Autodesk Fusion 360 part; units mm, degrees
sketch "Sketch1" plane through (0, 0, 0) normal (0, 0, 1) x (1, 0, 0)
  line L0 (0, 0) -> (42, 0)
  line L1 (42, 0) -> (42, 26)
  line L2 (42, 26) -> (0, 26)
  line L3 (0, 26) -> (0, 0)
  dimension "d1" = 42
  dimension "d2" = 26
extrude "Extrude1" add sketch "Sketch1" along normal blind 18
shell "Shell1" thickness 2 removed faces 1 at (14, 17.3333, 18)
extrude "Extrude2" cut 1 faces at (0, 17.3333, 12) along direction (-1, 0, 0) blind 10
extrude "Extrude3" cut 1 faces at (42, 8.6667, 6) along direction (1, 0, 0) blind 20
Could you check a few things on this model? Use its own coordinates, in mm. A direction names the side the tool comes from. Round coordinates to 2 decimals unless told otherwise and drop trailing zeros. Loops run counter-clockwise (first coordinate to the right, second up) from the corner with the lowest first, then second, coordinate; pieces in that order, holes last. Notation, with made-up numbers: (-28.75, -1.75) - (11.25, -1.75) arc R16 ccw to (11.25, 20.25) - close; hole circle Ø6 at (-26, 48). An arc over 180 degrees is marked (long way). Write item = value, one per line.
1) If we mould it in two halves opening along Y, with no side actions, what happens to faces 3 (the flat face through (2, 13, 10)), 4 (the flat face through (21, 24, 10)), 5 (the flat face through (21, 0, 9)), 6 (the flat face through (21, 26, 9))? For each: pulls with the +Y half, pulls with the -Y half, needs draft (parallel to the pull), parting line crosses it, or undercut.
Computed:
face_3 = undercut
face_4 = undercut
face_5 = pulls with the -Y half
face_6 = pulls with the +Y half
2) I'm going to push a flat-ended pin straight in: P1, Ø12, axis at x = 17, y = 15.5, coming from the +Z side. Where does the tip first touch, or does it pass through?
Computed:
P1 = 2
3) Imagine slicing it at A-A (z = 7). Please give me the cut outline in (x, y), and give its area (3 significant figures).
Computed:
outline = (0, 0) - (42, 0) - (42, 26) - (0, 26) - close; hole (2, 2) - (40, 2) - (40, 24) - (2, 24) - close
area = 256 mm2
4) Imagine slicing it at C-C (x = 10). Please give me the cut outline in (y, z), and give its area (3 significant figures).
Computed:
outline = (0, 0) - (26, 0) - (26, 18) - (24, 18) - (24, 2) - (2, 2) - (2, 18) - (0, 18) - close
area = 116 mm2
5) On a 3-axis mill with a long thin cutter (end or side, diameter ignored), from which of +Z, -Z, +X, -X, +Y, -Y can I reach the whole of each face in a straight line? I mean faces 1 (the flat face through (21, 13, 0)), 2 (the flat face through (40, 13, 10)). Say none if no direction works.
Computed:
face_1 = -Z, +X, -X, +Y, -Y
face_2 = +Z
6) I need wall thicknesses on line 1 along Y through (x, z) = (26.5, 17.25); line 2 along X through (y, z) = (15.5, 14); line 3 along Z through (x, y) = (23, 23.25). Which ranges of each line are inside material? Lowest first, please. Write a range as from..to.
Computed:
line_1 = 0..2, 24..26
line_2 = 0..2, 40..42
line_3 = 0..2
7) Imagine slicing it at B-B (y = 8.25). Please give me the cut outline in (x, z).
Computed:
outline = (0, 0) - (42, 0) - (42, 18) - (40, 18) - (40, 2) - (2, 2) - (2, 18) - (0, 18) - close
